Check sheet for the drawn part. Datum: minimum x, y, z corner. Units: mm. A direction names the side the tool comes from. Round coordinates to 2 decimals unless told otherwise and drop trailing zeros. Order: outer loops, then holes, each group sorted by start corner. A loop starts at its lowest first (then second) coordinate and runs counter-clockwise, first axis right, second up.
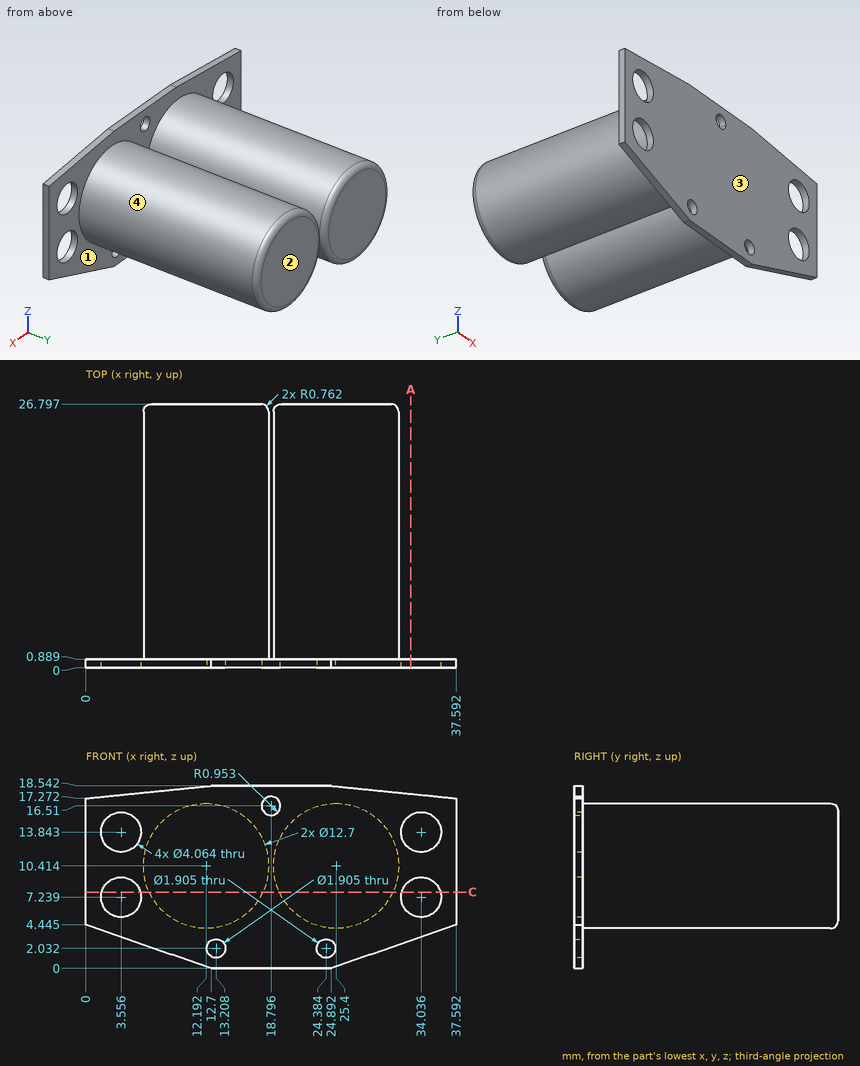
1) Draft check along X on the marked faces 1 and 2. Enter one of: pulls with the +X half, pulls with the -X half, needs draft (parallel to the pull), parting line crosses it, or undercut.
2) Sectioned sample at A-A on x = 33. Record the cut outline in (y, z) (1 decimal).
3) Scan lines: line 1 (Y direction, x = 30, z = 4); line 2 (Z direction, x = 12, y = 22); line 3 (X direction, y = 5, z = 4.75) (1 decimal). Record each from-to range of solid material in increasing order.
4) Gauge pin test, flat ends, axial feed: pin 1 (2.5 mm diameter, centred on x = 13.208, z = 2.032, fed in from +Y); pin 2 (10 mm diameter, centred on y = 7, z = 6.5, fed in from -X); pin 3 (3 mm diameter, centred on y = 8.5, z = 4.5, fed in from +X) (1 decimal); pin 4 (1.1 mm diameter, centred on x = 24.384, z = 2.032, fed in from -Y). Record the tip position at first contact, or that the pin passes through.
5) Sectioned sample at C-C on z = 7.75. Count the separate pieces of the cut face and the enclosed holes in it, and give its area (3 significant figures).
6) Set-up check for the marked faces 3 and 4: record each of +Z, -Z, +X, -X, +Y, -Y from which the full face is reachable in a straight line by a thin tool's end or side.
Values found:
1. face 1: undercut
1. face 2: needs draft
2. outline: (0, 2.8) - (0.9, 2.8) - (0.9, 5.5) - (0, 5.5) - close; (0, 9) - (0.9, 9) - (0.9, 12.1) - (0, 12.1) - close; (0, 15.6) - (0.9, 15.6) - (0.9, 17.7) - (0, 17.7) - close
3. line 1: y = 0 to 0.89
3. line 2: z = 4.07 to 16.76
3. line 3: x = 9.3 to 15.1, 22.5 to 28.3
4. pin 1: stops at y = 0.89
4. pin 2: stops at x = 5.84
4. pin 3: stops at x = 30
4. pin 4: passes through
5. separate pieces: 3
5. enclosed holes: 0
5. area: 623 mm2
6. face 3: +Z, -Z, +X, -X, -Y
6. face 4: +Y
